Read the model definition and answer for the solid it produces. Units are mm, in the model's axes. A direction names the side the tool comes from. Give positions to 0.01 mm unless a question says otherwise; leave off trailing zeros. Write each loop counter-clockwise with the first axis right and the second up, starting at its lowest first coordinate (ties: lowest second). Pieces come first, ordered by that corner, then holes.
```python
from build123d import *

# Parameters (mm, degrees)
SKETCH_R     = 4
SKETCH_R_2   = 2
PAD_DEPTH    = 12
POCKET_DEPTH = 6


with BuildPart() as part:
    # Sketch → Pad (new body)
    with BuildSketch(Plane.XY):
        with BuildLine():
            Line((-15, 17), (15, 17))
            Line((15, 17), (29.858612, 8.74036))
            ThreePointArc((29.858612, -8.74036), (35, 0), (29.858612, 8.74036))
            Line((15, -17), (29.858612, -8.74036))
            Line((15, -17), (-15, -17))
            Line((-15, -17), (-29.858612, -8.74036))
            ThreePointArc((-29.858612, 8.74036), (-35, 0), (-29.858612, -8.74036))
            Line((-15, 17), (-29.858612, 8.74036))
        make_face()
        with Locations((-25, 0)):
            Circle(SKETCH_R, mode=Mode.SUBTRACT)
        with Locations((25, 0)):
            Circle(SKETCH_R, mode=Mode.SUBTRACT)
        with Locations((-9, 12)):
            Circle(SKETCH_R_2, mode=Mode.SUBTRACT)
        with Locations((9, 12)):
            Circle(SKETCH_R_2, mode=Mode.SUBTRACT)
        with Locations((9, -12)):
            Circle(SKETCH_R_2, mode=Mode.SUBTRACT)
        with Locations((-9, -12)):
            Circle(SKETCH_R_2, mode=Mode.SUBTRACT)
    extrude(amount=PAD_DEPTH)

    # Sketch001 (on Face15 of Pad) → Pocket (cut)
    with BuildSketch(Plane(origin=(0, 0, 0), x_dir=(1, 0, 0), z_dir=(0, 0, -1))):
        Polygon((-28.839379, 6.65), (-32.678759, 0), (-28.839379, -6.65), (-21.160621, -6.65), (-17.321241, 0), (-21.160621, 6.65), align=None)
        Polygon((17.321241, 0), (21.160621, -6.65), (28.839379, -6.65), (32.678759, 0), (28.839379, 6.65), (21.160621, 6.65), align=None)
    extrude(amount=-POCKET_DEPTH, mode=Mode.SUBTRACT)


solid = part.part
```
Item 1: Find the intervals of material crossed by line 1 along Y through (x, z) = (-9, 3); line 2 along X through (y, z) = (5, 5.75); line 3 along X through (y, z) = (5.5, 2), in increasing order.
Result set:
line 1: y = -17 to -14, -10 to 10, 14 to 17
line 2: x = -33.66 to -29.79, -20.21 to 20.21, 29.79 to 33.66
line 3: x = -33.35 to -29.5, -20.5 to 20.5, 29.5 to 33.35
Item 2: Section D-D (z = 9.25) is taken. Write down the section's boundary in (x, y), and give its area (3 significant figures).
Result set:
outline: (-29.86, -8.74) - (-15, -17) - (15, -17) - (29.86, -8.74) arc R10 ccw to (29.86, 8.74) - (15, 17) - (-15, 17) - (-29.86, 8.74) arc R10 ccw to start; hole circle Ø8 at (-25, 0); hole circle Ø4 at (-9, -12); hole circle Ø4 at (-9, 12); hole circle Ø4 at (9, -12); hole circle Ø4 at (9, 12); hole circle Ø8 at (25, 0)
area: 1,760 mm2
Item 3: Section C-C (y = -12) is taken. Write down the section's boundary in (x, z).
Result set:
outline: (-23.99, 0) - (-11, 0) - (-11, 12) - (-23.99, 12) - close; (-7, 0) - (7, 0) - (7, 12) - (-7, 12) - close; (11, 0) - (23.99, 0) - (23.99, 12) - (11, 12) - close
Item 4: Determine the mould class of faces 3 (the flat face through (0, -17, 6)), 4 (the flat face through (0, 17, 6)), 5 (the flat face through (19.214, 3.278, 2.958)) for opening direction Y: pulls with the +Y half, pulls with the -Y half, needs draft (parallel to the pull), parting line crosses it, or undercut.
Result set:
face 3: pulls with the -Y half
face 4: pulls with the +Y half
face 5: undercut
Item 5: Section B-B (z = 2.75) is taken. Write down the section's boundary in (x, y).
Result set:
outline: (-29.86, -8.74) - (-15, -17) - (15, -17) - (29.86, -8.74) arc R10 ccw to (29.86, 8.74) - (15, 17) - (-15, 17) - (-29.86, 8.74) arc R10 ccw to start; hole (-32.68, 0) - (-28.84, -6.65) - (-21.16, -6.65) - (-17.32, 0) - (-21.16, 6.65) - (-28.84, 6.65) - close; hole circle Ø4 at (-9, -12); hole circle Ø4 at (-9, 12); hole circle Ø4 at (9, -12); hole circle Ø4 at (9, 12); hole (17.32, 0) - (21.16, -6.65) - (28.84, -6.65) - (32.68, 0) - (28.84, 6.65) - (21.16, 6.65) - close
Item 6: Each of these flat-tipped pins is pushed along its axis until it touches: pin 1 Ø1.8 at (x, z) = (26.5, 4) entering from +Y; pin 2 Ø5 at (x, z) = (-23.5, 4) entering from -Y; pin 3 Ø2 at (y, z) = (-8.5, 6) entering from -X. Where does it stop, or does it pass through?
Result set:
pin 1: stops at y = 11.11
pin 2: stops at y = -13.66
pin 3: stops at x = -31.61
Item 7: Section A-A (x = 9) is taken. Write down the section's boundary in (y, z), and give its area (3 significant figures).
Result set:
outline: (-17, 0) - (-14, 0) - (-14, 12) - (-17, 12) - close; (-10, 0) - (10, 0) - (10, 12) - (-10, 12) - close; (14, 0) - (17, 0) - (17, 12) - (14, 12) - close
area: 312 mm2
Item 8: Which of the six approach directions +Z, -Z, +X, -X, +Y, -Y give full straight-line access (tool end or side, diameter ignored) to faces 1 (the flat face through (25, -6.65, 3)), 2 (the cylindrical face through (-9, 14, 6))?
Result set:
face 1: -Z
face 2: +Z, -Z
